Source: CAD feature listing. Evaluate the final solid. Frame: model axes, mm. Face numbers are marked on the shaded views. A direction names the side the tool comes from. Round coordinates to 2 decimals unless told otherwise and drop trailing zeros. Write each loop counter-clockwise with the first axis right and the second up, starting at its lowest first coordinate (ties: lowest second). Pieces come first, ordered by that corner, then holes.
from build123d import *

# Parameters (mm, degrees)
BOSS_EXTRUDE1_DEPTH    = 32
SKETCH2_R              = 20
CUT_EXTRUDE1_DEPTH     = 33
BOSS_EXTRUDE2_DEPTH    = 18
F_16_0MM_DOWEL_SLOT1_D = 16


with BuildPart() as part:
    # Sketch1 → Boss-Extrude1 (new body)
    with BuildSketch(Plane.XY):
        with BuildLine():
            Line((-38, 0), (-38, -84))
            Line((-38, -84), (-16, -84))
            Line((-16, -84), (-16, -36))
            Line((-16, -36), (16, -36))
            Line((16, -36), (16, -84))
            Line((16, -84), (38, -84))
            Line((38, -84), (38, 0))
            ThreePointArc((38, 0), (0, 38), (-38, 0))
        make_face()
    extrude(amount=BOSS_EXTRUDE1_DEPTH)

    # Sketch2 → Cut-Extrude1 (cut, through all)
    with BuildSketch(Plane.XY.offset(32)):
        Circle(SKETCH2_R)
    extrude(amount=-CUT_EXTRUDE1_DEPTH, mode=Mode.SUBTRACT)

    # Sketch3 → Boss-Extrude2 (add)
    with BuildSketch(Plane.ZY.offset(38)):
        with BuildLine():
            Line((32, -84), (92, -84))
            ThreePointArc((92, -84), (108, -68), (92, -52))
            Line((92, -52), (32, -38))
            Line((32, -38), (32, -84))
        make_face()
    boss_extrude2 = extrude(amount=-BOSS_EXTRUDE2_DEPTH)

    # Mirror1: Boss-Extrude2 across plane
    add(boss_extrude2.mirror(Plane(origin=(0, 0, 0), x_dir=(0, 0, 1), z_dir=(1, 0, 0))))

    # Ø16.0mm Dowel Slot1 (through all)
    with Locations(Plane.ZY.offset(38)):
        with Locations((91.877349946, -68.13604901)):
            Hole(F_16_0MM_DOWEL_SLOT1_D / 2)


solid = part.part
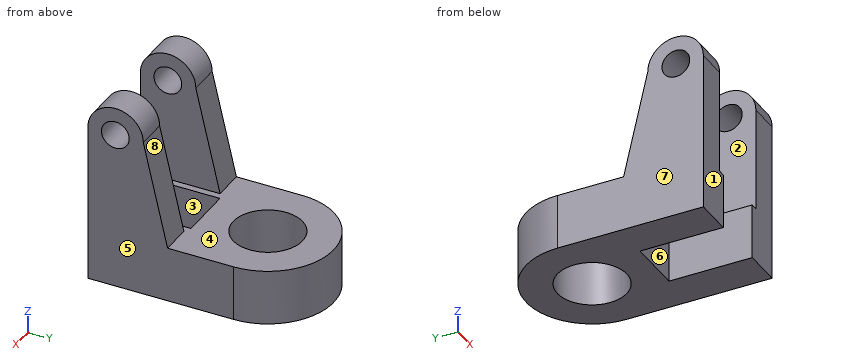
1) Section query C-C on z = 34. Return the cut outline in (x, y).
Taken from the geometry:
outline: (-38, -84) - (-20, -84) - (-20, -38.47) - (-38, -38.47) - close; (20, -84) - (38, -84) - (38, -38.47) - (20, -38.47) - close
2) Contact query for a flat-ended pin moving along its axis: P1, Ø8, axis at x = 10, y = -16, coming from the +Z side. Output: stop coordinate, or through.
Taken from the geometry:
P1: stops at z = 32
3) Section query D-D on x = 22.5. Return the cut outline in (y, z).
Taken from the geometry:
outline: (-84, 0) - (30.62, 0) - (30.62, 32) - (-38, 32) - (-52, 92) arc R16 ccw to (-84, 92) - close; hole circle Ø16 at (-68.14, 91.88)
4) Section query A-A on x = 0. Return the cut outline in (y, z), then the cut area to 3 significant figures.
Taken from the geometry:
outline: (-36, 0) - (-20, 0) - (-20, 32) - (-36, 32) - close; (20, 0) - (38, 0) - (38, 32) - (20, 32) - close
area: 1,090 mm2
5) Section query B-B on y = -58. Return the cut outline in (x, z).
Taken from the geometry:
outline: (-38, 0) - (-16, 0) - (-16, 32) - (-20, 32) - (-20, 104.49) - (-38, 104.49) - close; (16, 0) - (38, 0) - (38, 104.49) - (20, 104.49) - (20, 32) - (16, 32) - close
6) Pull-direction query (X, two-part tool) for the marked faces 5, 6, 7 and 8; classes: released by +X, released by -X, zero draft, split by the parting line, or undercut.
Taken from the geometry:
face 5: released by +X
face 6: undercut
face 7: released by -X
face 8: zero draft
7) Material intervals for line 1 (X direction, y = -61, z = 31); line 2 (X direction, y = -53, z = 75.5); line 3 (Y direction, x = 0, z = 21.5), sorted ascending.
Taken from the geometry:
line 1: x = -38 to -16, 16 to 38
line 2: x = -38 to -20, 20 to 38
line 3: y = -36 to -20, 20 to 38
8) Reachability of the marked faces 1, 2, 3 and 4 from +Z, -Z, +X, -X, +Y, -Y: full face, straight path, thin tool, end or side. Return the list, or none.
Taken from the geometry:
face 1: +Z, -Z, +X, -X, -Y
face 2: +Z, +Y, -Y
face 3: +Z, -Z, -Y
face 4: +Z, +Y
